Could you check a few things on this model? Use its own coordinates, in mm. Face numbers are marked on the shaded views. A direction names the side the tool comes from. Give positions to 0.01 mm unless a question says otherwise; leave off trailing zeros. Order: outer loops, then holes, each group sorted by start corner. A loop starts at its lowest first (then second) coordinate and runs counter-clockwise, first axis right, second up. Notation, with made-up numbers: (33.5, 24.25) -> (54.5, 24.25) arc R18 ccw to (54.5, 41.25) -> close; hole circle Ø11 at (-38, 89). An arc over 180 degrees is marked (long way). Write each question's results on one line, items separated by ' | '.
```python
from build123d import *

# Parameters (mm, degrees)
F1_DEPTH = 30
F3_DEPTH = 30.001
F4_R     = 5
F5_R     = 4
F6_DEPTH = 43.001


with BuildPart() as f1:
    # F0 (on Right) → F1 (new body)
    with BuildSketch(Plane.YZ):
        Polygon((-12, 40), (-15, 40), (-15, -3), (15, -3), (15, 40), (12, 40), (12, 0), (-12, 0), align=None)
    extrude(amount=F1_DEPTH)

    # F2 (on face) → F3 (cut, through all)
    with BuildSketch(Plane(origin=(0, 15, 0), x_dir=(-1, 0, 0), z_dir=(0, 1, 0))):
        with BuildLine():
            ThreePointArc((-15, 22), (-10.757359, 23.757359), (-9, 28))
            ThreePointArc((-9, 28), (-10.757359, 32.242641), (-15, 34))
            Line((-15, 34), (-15, 22))
        make_face()
        with BuildLine():
            Line((-15, 22), (-15, 34))
            ThreePointArc((-15, 34), (-21, 28), (-15, 22))
        make_face()
    extrude(amount=-F3_DEPTH, mode=Mode.SUBTRACT)

    # F4
    f4_edges = [f1.edges().sort_by_distance(p)[0] for p in [
        (0, 13.5, 40),
        (0, -13.5, 40),
        (30, 13.5, 40),
        (30, -13.5, 40),
    ]]
    fillet(f4_edges, radius=F4_R)

    # F5 (on face) → F6 (cut, through all)
    with BuildSketch(Plane(origin=(0, 0, -3), x_dir=(1, 0, 0), z_dir=(0, 0, -1))):
        with Locations((15, 0)):
            Circle(F5_R)
    extrude(amount=-F6_DEPTH, mode=Mode.SUBTRACT)


solid = f1.part
```
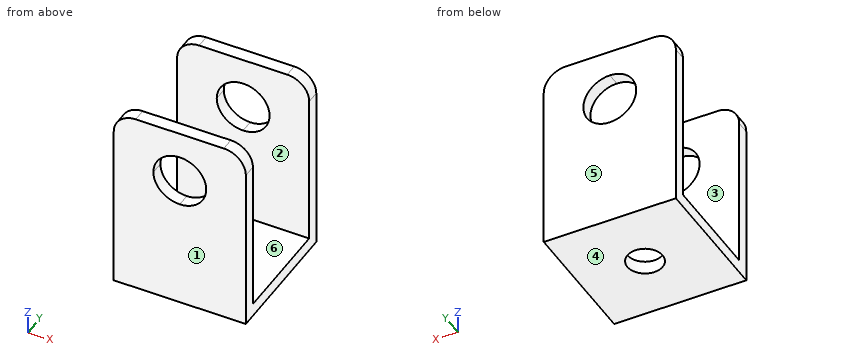
Q1. I'm going to push a flat-ended pin straight in: pin 1 Ø4 at (x, y) = (13.5, 5.5) entering from +Z. Where does the tip first touch, or does it pass through?
Here are the results:
pin 1: stops at z = 0
Q2. Suppose I cut it at D-D on z = 22.5. Please give me the cut outline in (x, y).
Here are the results:
outline: (0, -15) -> (12.6, -15) -> (12.6, -12) -> (0, -12) -> close; (0, 12) -> (12.6, 12) -> (12.6, 15) -> (0, 15) -> close; (17.4, -15) -> (30, -15) -> (30, -12) -> (17.4, -12) -> close; (17.4, 12) -> (30, 12) -> (30, 15) -> (17.4, 15) -> close
Q3. Suppose I cut it at C-C on x = 23.25. Please give me the cut outline in (y, z), and give its area (3 significant figures).
Here are the results:
outline: (-15, -3) -> (15, -3) -> (15, 40) -> (12, 40) -> (12, 0) -> (-12, 0) -> (-12, 40) -> (-15, 40) -> close | area: 330 mm²
Q4. Suppose I cut it at B-B on z = 0.5. Please give me the cut outline in (x, y).
Here are the results:
outline: (0, -15) -> (30, -15) -> (30, -12) -> (0, -12) -> close; (0, 12) -> (30, 12) -> (30, 15) -> (0, 15) -> close
Q5. Thinking about a two-plate mould opening in Y: for the marked faces 3, 4, 5 and 6, which applies, +Y half, -Y half, draft (parallel to the pull), parting line (faces both ways), or undercut?
Here are the results:
face 3: undercut | face 4: draft | face 5: +Y half | face 6: undercut
Q6. I need wall thicknesses on line 1 along Y through (x, z) = (26.5, 13); line 2 along X through (y, z) = (0, -2.3); line 3 along Y through (x, z) = (15, -0.8). Which ranges of each line are inside material? Lowest first, please.
Here are the results:
line 1: y = -15 to -12, 12 to 15 | line 2: x = 0 to 11, 19 to 30 | line 3: y = -15 to -4, 4 to 15
Q7. For the marked faces 1 and 2, which set-ups out of +Z, -Z, +X, -X, +Y, -Y let a thin tool reach every point of the face, with its end or its side?
Here are the results:
face 1: +Z, -Z, +X, -X, -Y | face 2: +Z, +X, -X
Q8. Suppose I cut it at A-A on y = 0. Please give me the cut outline in (x, z), and give its area (3 significant figures).
Here are the results:
outline: (0, -3) -> (11, -3) -> (11, 0) -> (0, 0) -> close; (19, -3) -> (30, -3) -> (30, 0) -> (19, 0) -> close | area: 66.0 mm²
